from build123d import *

# Parameters (mm, degrees)
BOSS_EXTRUDE1_DEPTH = 277.475
CUT_EXTRUDE1_REACH  = 284.517
SKETCH2_R           = 2.5


with BuildPart() as part:
    # Sketch1 → Boss-Extrude1 (new body)
    with BuildSketch(Plane.XY):
        Polygon((-37.629508919, -38.824877845), (-13.751817824, 56.943310339), (-16.832506755, 57.711412357), (-40.71019785, -38.056775826), align=None)
    extrude(amount=BOSS_EXTRUDE1_DEPTH)

    # Sketch2 → Cut-Extrude1 (cut, up to next)
    with BuildSketch(Plane(origin=(-26.313608582, 6.560719475, 0), x_dir=(0, 0, -1), z_dir=(0.9702957262759973, -0.24192189559966462, 0)), mode=Mode.PRIVATE) as cut_extrude1_sk1:
        with Locations(Location((-207.475, 2.616835031, 0), (0, 0, 90))):
            Circle(SKETCH2_R)
    cut_extrude1_tool1 = extrude(cut_extrude1_sk1.sketch, amount=-CUT_EXTRUDE1_REACH, mode=Mode.PRIVATE) & part.part
    # Sketch2 → Cut-Extrude1 (cut, up to next)
    with BuildSketch(Plane(origin=(-26.313608582, 6.560719475, 0), x_dir=(0, 0, -1), z_dir=(0.9702957262759973, -0.24192189559966462, 0)), mode=Mode.PRIVATE) as cut_extrude1_sk2:
        with Locations(Location((-70, 2.616835031, 0), (0, 0, 90))):
            Circle(SKETCH2_R)
    cut_extrude1_tool2 = extrude(cut_extrude1_sk2.sketch, amount=-CUT_EXTRUDE1_REACH, mode=Mode.PRIVATE) & part.part
    add(cut_extrude1_tool1.solids().sort_by_distance((-25.680539, 9.099823, 207.475))[0], mode=Mode.SUBTRACT)
    add(cut_extrude1_tool2.solids().sort_by_distance((-25.680539, 9.099823, 70))[0], mode=Mode.SUBTRACT)


solid = part.part
The listing builds one solid part. Answer for the finished solid, in the listing's coordinates (mm). Give positions to 0.01 mm unless a question says otherwise; leave off trailing zeros. Write each loop counter-clockwise with the first axis right and the second up, starting at its lowest first coordinate (ties: lowest second). Pieces come first, ordered by that corner, then holes.
Item 1: Section A-A, the plane z = 139 is taken. Write down the section's boundary in (x, y), plus the area to 3 significant figures.
Item 2: Section B-B, the plane x = -21.75 is taken. Write down the section's boundary in (y, z) (3 decimals).
Item 3: Flat-ended cylindrical pins translate along their axes: P1, Ø1, axis at x = -18, y = 31.5, coming from the -Z side; P2, Ø5, axis at y = 41, z = 115, coming from the -X side; P3, Ø8, axis at y = -4, z = 43.5, coming from the -X side; P4, Ø1.5, axis at y = 17, z = 31, coming from the +X side. Find the tip coordinate at first contact, or state that the pin passes through.
Item 4: Find the intervals of material crossed by line 1 along X through (y, z) = (-22, 13); line 2 along X through (y, z) = (-16, 77.5), in increasing order.
Item 5: Determine the mould class of faces 1 (the cylindrical face through (-27.33, 8.95, 67.56)), 2 (the flat face through (-25.858, 8.389, 136.795)), 3 (the flat face through (-27, 10, 0)) for opening direction Z: released by +Z, released by -Z, zero draft, split by the parting line, or undercut.
Completed:
1. outline: (-40.71, -38.06) - (-37.63, -38.82) - (-13.75, 56.94) - (-16.83, 57.71) - close
1. area: 313 mm2
2. outline: (24.864, 0) - (37.988, 0) - (37.988, 277.475) - (24.864, 277.475) - close
3. P1: passes through
3. P2: stops at x = -21.62
3. P3: stops at x = -33.22
3. P4: stops at x = -23.52
4. line 1: x = -36.71 to -33.43
4. line 2: x = -35.21 to -31.94
5. face 1: undercut
5. face 2: zero draft
5. face 3: released by -Z
